Work out the finished part from the listing and answer in its coordinate system (mm). A direction names the side the tool comes from. Round coordinates to 2 decimals unless told otherwise and drop trailing zeros. Write each loop counter-clockwise with the first axis right and the second up, starting at its lowest first coordinate (ties: lowest second). Pieces come first, ordered by that corner, then holes.
1. Flat-ended cylindrical pins translate along their axes: pin 1 Ø3 at (x, y) = (-0.5, -6) entering from -Z; pin 2 Ø1.8 at (x, y) = (0.5, 4) entering from -Z; pin 3 Ø3 at (x, z) = (-14, 7.5) entering from +Y; pin 4 Ø12 at (x, y) = (12.5, -16.5) entering from -Z. Find the tip coordinate at first contact, or state that the pin passes through.
2. Straight lines are drawn through the part: probe 1 along Y at (x, z) = (0, 6.6); probe 2 along X at (y, z) = (10.7, 5.5); probe 3 along X at (y, z) = (-14.5, 7). For each, find the intervals that lie inside material, in ascending order.
3. Determine the mould class of faces 6 (the face through (0.065, 4.496, 6.465)), 7 (the face through (0, -25, 10)), 8 (the face through (-12, 11, 5)) for opening direction Y: pulls with the +Y half, pulls with the -Y half, needs draft (parallel to the pull), parting line crosses it, or undercut.
4. A tool of negligible diameter and unlimited length cuts with its end or side. For faces 1 (the face through (-13, 10, 5)), 2 (the face through (-8, 19, 5)), 3 (the face through (0, 3, 4)), 4 (the face through (0, 4, 9)), 5 (the face through (8, 19, 5)), from which of +Z, -Z, +X, -X, +Y, -Y can it reach the whole face along a straight path? Write none if from no direction.
5. Find section C-C (z = 3.25). Write down the section's boundary in (x, y), and give its area (3 significant figures).
6. Find section A-A (z = 7.5). Write down the section's boundary in (x, y).
7. Find section D-D (x = -5). Write down the section's boundary in (y, z), and give its area (3 significant figures).
8. Find section B-B (y = -11). Write down the section's boundary in (x, z).
```python
from build123d import *

# Parameters (mm, degrees)
BOSS_EXTRU_1_DEPTH      = 9
ESQUISSE2_W             = 16
ESQUISSE2_H             = 52
BOSS_EXTRU_2_DEPTH      = 2
ESQUISSE5_R             = 1.75
BOSS_EXTRU_5_DEPTH      = 5
ESQUISSE6_R             = 0.5
ENL_V_MAT_EXTRU_1_DEPTH = 5
ESQUISSE11_W            = 11
ESQUISSE11_H            = 2
BOSS_EXTRU_6_DEPTH      = 10
ESQUISSE12_R            = 0.5
ENL_V_MAT_EXTRU_2_DEPTH = 38


with BuildPart() as part:
    # Esquisse1 → Boss.-Extru.1 (new body)
    with BuildSketch(Plane.XY):
        Polygon((-6, -25), (-6, 25), (6, 25), (6, -25), (8, -25), (8, 27), (-8, 27), (-8, -25), align=None)
    extrude(amount=BOSS_EXTRU_1_DEPTH)

    # Esquisse2 → Boss.-Extru.2 (add)
    with BuildSketch(Plane.XY.offset(9)):
        with Locations((0, 1)):
            Rectangle(ESQUISSE2_W, ESQUISSE2_H)
    extrude(amount=BOSS_EXTRU_2_DEPTH)

    # Esquisse5 → Boss.-Extru.5 (add)
    with BuildSketch(Plane(origin=(0, 0, 9), x_dir=(-1, 0, 0), z_dir=(0, 0, -1))):
        with Locations((0, 4)):
            Circle(ESQUISSE5_R)
    extrude(amount=BOSS_EXTRU_5_DEPTH)

    # Esquisse6 → Enlèv. mat.-Extru.1 (cut)
    with BuildSketch(Plane(origin=(0, 0, 4), x_dir=(-1, 0, 0), z_dir=(0, 0, -1))):
        with Locations((0, 4)):
            Circle(ESQUISSE6_R)
    extrude(amount=-ENL_V_MAT_EXTRU_1_DEPTH, mode=Mode.SUBTRACT)

    # Esquisse11 → Boss.-Extru.6 (add)
    with BuildSketch(Plane.ZY.offset(8)):
        with Locations((5.5, 11)):
            Rectangle(ESQUISSE11_W, ESQUISSE11_H)
    boss_extru_6 = extrude(amount=BOSS_EXTRU_6_DEPTH)

    # Esquisse12 → Enlèv. mat.-Extru.2 (cut, through all)
    with BuildSketch(Plane(origin=(0, 12, 0), x_dir=(1, 0, 0), z_dir=(0, 1, 0))):
        with Locations((-12, -5.5)):
            Circle(ESQUISSE12_R)
    enl_v_mat_extru_2 = extrude(amount=-ENL_V_MAT_EXTRU_2_DEPTH, mode=Mode.SUBTRACT)

    # Symétrie1: Boss.-Extru.6, Enlèv. mat.-Extru.2 across plane
    add(boss_extru_6.mirror(Plane(origin=(0, 0, 0), x_dir=(0, 0, 1), z_dir=(1, 0, 0))))
    add(enl_v_mat_extru_2.mirror(Plane(origin=(0, 0, 0), x_dir=(0, 0, 1), z_dir=(1, 0, 0))), mode=Mode.SUBTRACT)


solid = part.part
```
Worked answers:
1. pin 1: stops at z = 9
1. pin 2: stops at z = 4
1. pin 3: stops at y = 12
1. pin 4: stops at z = 0
2. probe 1: y = 2.25 to 3.5, 4.5 to 5.75, 25 to 27
2. probe 2: x = -18 to -12.5, -11.5 to -6, 6 to 11.5, 12.5 to 18
2. probe 3: x = -8 to -6, 6 to 8
3. face 6: undercut
3. face 7: pulls with the -Y half
3. face 8: needs draft
4. face 1: +Z, -Z, -X, -Y
4. face 2: +Z, -Z, -X, +Y
4. face 3: -Z, -Y
4. face 4: -Z
4. face 5: +Z, -Z, +X, +Y
5. outline: (-18, 10) - (-8, 10) - (-8, -25) - (-6, -25) - (-6, 25) - (6, 25) - (6, -25) - (8, -25) - (8, 10) - (18, 10) - (18, 12) - (8, 12) - (8, 27) - (-8, 27) - (-8, 12) - (-18, 12) - close
5. area: 272 mm2
6. outline: (-18, 10) - (-8, 10) - (-8, -25) - (-6, -25) - (-6, 25) - (6, 25) - (6, -25) - (8, -25) - (8, 10) - (18, 10) - (18, 12) - (8, 12) - (8, 27) - (-8, 27) - (-8, 12) - (-18, 12) - close; circle Ø3.5 at (0, 4); hole circle Ø1 at (0, 4)
7. outline: (-25, 9) - (25, 9) - (25, 0) - (27, 0) - (27, 11) - (-25, 11) - close
7. area: 122 mm2
8. outline: (-8, 0) - (-6, 0) - (-6, 9) - (6, 9) - (6, 0) - (8, 0) - (8, 11) - (-8, 11) - close
